```python
from build123d import *

# Parameters (mm, degrees)
EXTRUDE_THIN1_DEPTH = 7.5
SKETCH4_W           = 106
SKETCH4_H           = 15
BOSS_EXTRUDE1_DEPTH = 9
SKETCH5_R           = 4.5
CUT_EXTRUDE1_DEPTH  = 124.029468015


with BuildPart() as part:
    # Sketch1 → Extrude-Thin1 (new, symmetric)
    with BuildSketch(Plane.XY):
        Polygon((-50, 0), (-50, -50), (50, -50), (50, 0), (53, 0), (53, -53), (-53, -53), (-53, 0), align=None)
    extrude(amount=EXTRUDE_THIN1_DEPTH, both=True)

    # Sketch4 → Boss-Extrude1 (add)
    with BuildSketch(Plane.XZ.offset(53)):
        Rectangle(SKETCH4_W, SKETCH4_H)
    extrude(amount=BOSS_EXTRUDE1_DEPTH)

    # Sketch5 → Cut-Extrude1 (cut, through all)
    with BuildSketch(Plane(origin=(53, 0, 0), x_dir=(0, 0, -1), z_dir=(1, 0, 0))):
        with Locations(Location((0, -56, 0), (0, 0, 90))):
            Circle(SKETCH5_R)
    extrude(amount=-CUT_EXTRUDE1_DEPTH, mode=Mode.SUBTRACT)


solid = part.part
```
The model under review builds one solid part; all positions refer to its coordinate system, in mm. A direction names the side the tool comes from. Give positions to 0.01 mm unless a question says otherwise; leave off trailing zeros. Write each loop counter-clockwise with the first axis right and the second up, starting at its lowest first coordinate (ties: lowest second). Pieces come first, ordered by that corner, then holes. Notation, with made-up numbers: (3.25, 65.5) - (48.25, 65.5) arc R18 cw to (48.25, 93.5) - close; hole circle Ø8 at (-17.5, 82). An arc over 180 degrees is marked (long way). Answer in a Markdown table with one row per item. Add a question column.
1. We need section C-C on x = 3. Write out the cut boundary in (y, z).
2. Draft analysis for pull direction Y (two halves, no side actions). For faces 3 (the flat face through (4, -52, 7.5)), 4 (the flat face through (-52, 0, 0)), 5 (the cylindrical face through (0.742, -51.708, 1.352)), state which applies: +Y half, -Y half, draft (parallel to the pull), parting line (faces both ways), or undercut.
3. Wall thickness on line 1 along X through (y, z) = (-4.5, -4.5); line 2 along Z through (x, y) = (11.5, -56); line 3 along Y through (x, z) = (-2.5, 3): over which ranges is each line inside the solid? List them lowest first. Write a range as [from, to].
4. We need section A-A on y = -34.5. Write out the cut boundary in (x, z), then the cut area to 3 significant figures.
5. We need section D-D on z = -6. Write out the cut boundary in (x, y).
6. Insertion check: P1, Ø3, axis at x = 13, z = 2, coming from the +Y side. The pin has a flat end and moves straight along its axis. Give the tip position at first contact, or say it passes through.
7. We need section B-B on z = 0. Write out the cut boundary in (x, y).
8. Tool access review of faces 1 (the flat face through (-50, -25, 0)), 2 (the flat face through (51, 0, 0)): name each direction out of +Z, -Z, +X, -X, +Y, -Y from which nothing blocks a thin tool from reaching the whole face with its end or side.
Ans:
| question | item | result |
|---|---|---|
| 1 | outline | (-62, -7.5) - (-50, -7.5) - (-50, 7.5) - (-62, 7.5) - close; hole circle Ø9 at (-56, 0) |
| 2 | face 3 | draft |
| 2 | face 4 | +Y half |
| 2 | face 5 | undercut |
| 3 | line 1 | x = [-53, -50], [50, 53] |
| 3 | line 2 | z = [-7.5, -4.5], [4.5, 7.5] |
| 3 | line 3 | y = [-62, -59.35], [-52.65, -50] |
| 4 | outline | (-53, -7.5) - (-50, -7.5) - (-50, 7.5) - (-53, 7.5) - close; (50, -7.5) - (53, -7.5) - (53, 7.5) - (50, 7.5) - close |
| 4 | area | 90.0 mm^2 |
| 5 | outline | (-53, -62) - (53, -62) - (53, 0) - (50, 0) - (50, -50) - (-50, -50) - (-50, 0) - (-53, 0) - close |
| 6 | P1 | stops at y = -50 |
| 7 | outline | (-53, -62) - (53, -62) - (53, -60.5) - (-53, -60.5) - close; (-53, -51.5) - (53, -51.5) - (53, 0) - (50, 0) - (50, -50) - (-50, -50) - (-50, 0) - (-53, 0) - close |
| 8 | face 1 | +Z, -Z, +Y |
| 8 | face 2 | +Z, -Z, +X, -X, +Y |
